Geometry: final body of the model. Coordinates: model frame, mm. A direction names the side the tool comes from. Coordinates: 2 decimals unless noted, no trailing zeros. Order: outer loops, then holes, each group sorted by start corner. A loop starts at its lowest first (then second) coordinate and runs counter-clockwise, first axis right, second up. Notation, with made-up numbers: M 84.25,71.5 L 106.25,71.5 A24 ccw 106.25,93.5 Z; hole C -7,70 d11. An arc over 180 degrees is marked long. Write item = value, one per line.
from build123d import *

# Parameters (mm, degrees)
F1_DEPTH = 25.4
F2_DEPTH = 25.4
F3_DEPTH = 12.7


# Not quite as in the source:
# - a feature names something its author has since deleted; it is built from what else it names


with BuildPart() as f1:
    # F0 (on Front) → F1 (new body, symmetric)
    with BuildSketch(Plane.XZ):
        Polygon((0, 38.1), (0, 0), (76.2, 0), (76.2, 12.7), (50.8, 12.7), (50.8, 25.4), (25.4, 25.4), (25.4, 50.8), (12.7, 50.8), align=None)
    extrude(amount=F1_DEPTH, both=True)

    # F0 (on Front) → F2 (join, symmetric)
    with BuildSketch(Plane.XZ):
        Polygon((38.1, 50.8), (25.4, 50.8), (25.4, 25.4), (50.8, 25.4), (50.8, 38.1), (38.1, 38.1), align=None)
    extrude(amount=F2_DEPTH, both=True)

    # F0 (on Front) → F3 (join, symmetric)
    with BuildSketch(Plane.XZ):
        Polygon((38.1, 50.8), (25.4, 50.8), (25.4, 25.4), (50.8, 25.4), (50.8, 38.1), (38.1, 38.1), align=None)
    extrude(amount=F3_DEPTH, both=True)


solid = f1.part
1) Line query: L1, parallel to X at y = -3, z = 17; L2, parallel to Z at x = 69.5, y = 23; L3, parallel to Z at x = 48.5, y = -23. Output: solid intervals per line, ascending.
Numbers:
L1 = 0 to 50.8
L2 = 0 to 12.7
L3 = 0 to 38.1
2) Section B-B, the plane x = 8.5. Return loops of the section in (y, z), and give its area (3 significant figures).
Numbers:
outline = M -25.4,0 L 25.4,0 L 25.4,46.6 L -25.4,46.6 Z
area = 2,370 mm²
3) Section A-A, the plane y = 4. Return loops of the section in (x, z).
Numbers:
outline = M 0,0 L 76.2,0 L 76.2,12.7 L 50.8,12.7 L 50.8,38.1 L 38.1,38.1 L 38.1,50.8 L 12.7,50.8 L 0,38.1 Z
4) Section C-C, the plane z = 16. Return loops of the section in (x, y).
Numbers:
outline = M 0,-25.4 L 50.8,-25.4 L 50.8,25.4 L 0,25.4 Z
5) Pin query (flat end, axial travel): pin 1 (7.5 mm diameter, centred on x = 57.5, y = -9, fed in from +Z); pin 2 (8 mm diameter, centred on y = 14.5, z = 30.5, fed in from +X); pin 3 (4 mm diameter, centred on x = 42, y = 11.5, fed in from +Z). Return the tip coordinate at first contact, or that it passes through.
Numbers:
pin_1 = 12.7
pin_2 = 50.8
pin_3 = 38.1
6) Set-up query: faces 1 (the face through (0, 0, 19)), 2 (the face through (50.8, 0, 25)). Return all of +Z, -Z, +X, -X, +Y, -Y with unobstructed straight access to the full face (end or side cutting, diameter ignored); none if empty.
Numbers:
face_1 = +Z, -Z, -X, +Y, -Y
face_2 = +Z, +X, +Y, -Y
